For this review, use the dimensioned drawing (mm, ordinates from the lowest corner) and the shaded views. Coordinates: 2 decimals unless noted, no trailing zeros. Order: outer loops, then holes, each group sorted by start corner. A loop starts at its lowest first (then second) coordinate and runs counter-clockwise, first axis right, second up. Notation, with made-up numbers: (34, 14.25) -> (68, 14.25) arc R20 ccw to (68, 32.25) -> close; hole circle Ø9 at (11.5, 63.25). An arc over 180 degrees is marked (long way). Return JSON: item names as keys, results as strings. Group by question number.
Item 1: Take a section at B-B (x = 177.5). Write out the cut boundary in (y, z), then the cut area to 3 significant figures.
Item 2: Take a section at A-A (z = 5). Write out the cut boundary in (x, y).
Item 3: For line 1 along Z through (x, y) = (22.5, 1.6); line 2 along X through (y, z) = (1.95, 5); line 3 along Z through (x, y) = (135.56, 2.05), list the stretches that pass through material, from the lowest coordinate up.
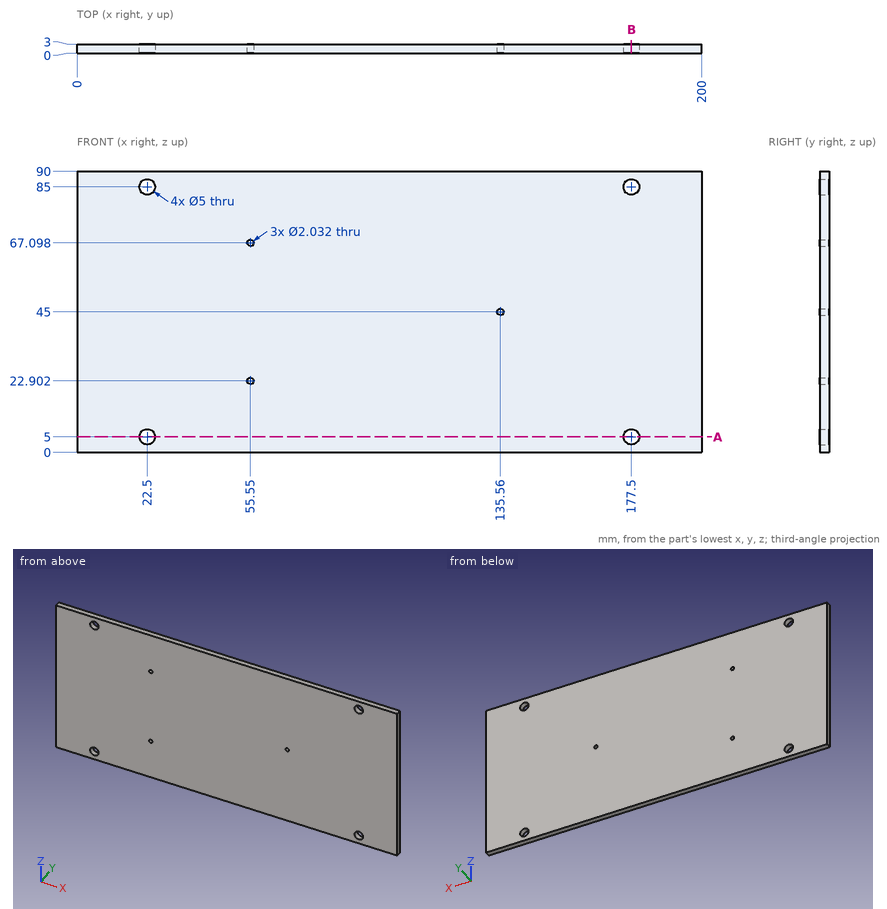
Findings below:
{
 "1": {"outline": "(0, 0) -> (3, 0) -> (3, 2.5) -> (0, 2.5) -> close; (0, 7.5) -> (3, 7.5) -> (3, 82.5) -> (0, 82.5) -> close; (0, 87.5) -> (3, 87.5) -> (3, 90) -> (0, 90) -> close", "area": "240 mm2"},
 "2": {"outline": "(0, 0) -> (20, 0) -> (20, 3) -> (0, 3) -> close; (25, 0) -> (175, 0) -> (175, 3) -> (25, 3) -> close; (180, 0) -> (200, 0) -> (200, 3) -> (180, 3) -> close"},
 "3": {"line 1": "z = 0 to 2.5, 7.5 to 82.5, 87.5 to 90", "line 2": "x = 0 to 20, 25 to 175, 180 to 200", "line 3": "z = 0 to 43.98, 46.02 to 90"}
}
